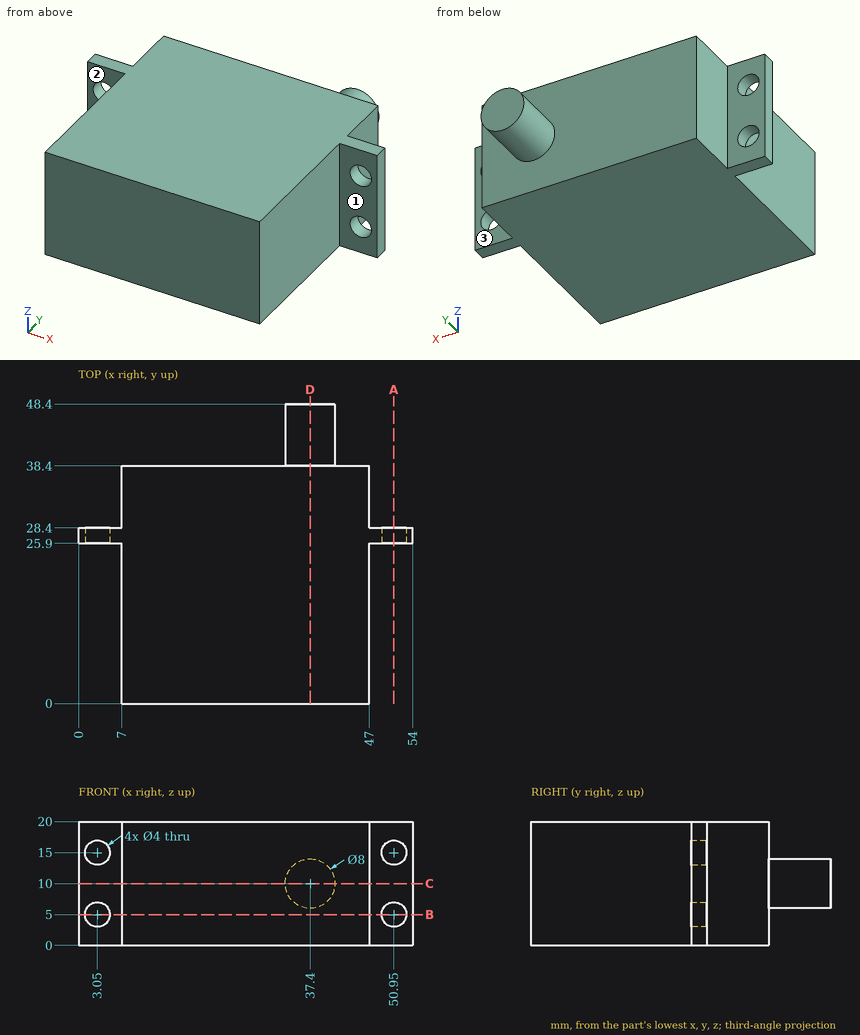
Verification items for this drawing (mm, ordinates from the low corner). A direction names the side the tool comes from. Give positions to 0.01 mm unless a question says otherwise; leave off trailing zeros. Write each loop counter-clockwise with the first axis right and the second up, starting at its lowest first coordinate (ties: lowest second). Pieces come first, ordered by that corner, then holes. Notation, with made-up numbers: (22, 71.5) -> (30, 71.5) arc R11 ccw to (30, 92.5) -> close; hole circle Ø2 at (-36.75, -0.75). An arc over 180 degrees is marked (long way). Use CSV: the item, a comma, the result in double quotes. Start each with the question number.
Q1. Cross-section at D-D on x = 37.4. Enter the section's corners in (y, z), and give its area (3 significant figures).
Q2. Tool access check on the marked faces 1, 2 and 3. Record the directions out of +Z, -Z, +X, -X, +Y, -Y that give a thin tool (end or side, any length) a straight path to the whole face; none if there is none.
Q3. Cross-section at B-B on z = 5. Enter the section's corners in (x, y), and give its area (3 significant figures).
Q4. Scan lines: line 1 along Z through (x, y) = (3, 27); line 2 along X through (y, z) = (27.1, 5); line 3 along Z through (x, y) = (50, 27). Record each from-to range of solid material in increasing order.
Q5. Cross-section at A-A on x = 50.95. Enter the section's corners in (y, z), and give its area (3 significant figures).
Q6. Depth check by flat-ended pin: P1, Ø1, axis at x = 19, y = 12.5, coming from the -Z side; P2, Ø2, axis at x = 2.5, z = 6, coming from the -Y side; P3, Ø4, axis at y = 18, z = 4.5, coming from the +X side; P4, Ø7.5, axis at x = 50.5, z = 8, coming from the +Y side. Enter the tip coordinate at first touch or a pass-through.
Q7. Cross-section at C-C on z = 10. Enter the section's corners in (x, y).
Working result:
1,outline,"(0, 0) -> (38.4, 0) -> (38.4, 6) -> (48.4, 6) -> (48.4, 14) -> (38.4, 14) -> (38.4, 20) -> (0, 20) -> close"
1,area,"848 mm^2"
2,face 1,"+Z, -Z, +X, -Y"
2,face 2,"+Z, -Z, -X, -Y"
2,face 3,"+Z, -Z, +X, +Y"
3,outline,"(0, 25.9) -> (1.05, 25.9) -> (1.05, 28.4) -> (0, 28.4) -> close; (5.05, 25.9) -> (7, 25.9) -> (7, 0) -> (47, 0) -> (47, 25.9) -> (48.95, 25.9) -> (48.95, 28.4) -> (47, 28.4) -> (47, 38.4) -> (7, 38.4) -> (7, 28.4) -> (5.05, 28.4) -> close; (52.95, 25.9) -> (54, 25.9) -> (54, 28.4) -> (52.95, 28.4) -> close"
3,area,"1,550 mm^2"
4,line 1,"z = 0 to 3, 7 to 13, 17 to 20"
4,line 2,"x = 0 to 1.05, 5.05 to 48.95, 52.95 to 54"
4,line 3,"z = 0 to 3.24, 6.76 to 13.24, 16.76 to 20"
5,outline,"(25.9, 0) -> (28.4, 0) -> (28.4, 3) -> (25.9, 3) -> close; (25.9, 7) -> (28.4, 7) -> (28.4, 13) -> (25.9, 13) -> close; (25.9, 17) -> (28.4, 17) -> (28.4, 20) -> (25.9, 20) -> close"
5,area,"30.0 mm^2"
6,P1,"stops at z = 0"
6,P2,"stops at y = 25.9"
6,P3,"stops at x = 47"
6,P4,"stops at y = 38.4"
7,outline,"(0, 25.9) -> (7, 25.9) -> (7, 0) -> (47, 0) -> (47, 25.9) -> (54, 25.9) -> (54, 28.4) -> (47, 28.4) -> (47, 38.4) -> (41.4, 38.4) -> (41.4, 48.4) -> (33.4, 48.4) -> (33.4, 38.4) -> (7, 38.4) -> (7, 28.4) -> (0, 28.4) -> close"
